from build123d import *

# Parameters (mm, degrees)
SKETCH1_R           = 14.9
BOSS_EXTRUDE1_DEPTH = 3
SKETCH2_R           = 7
CUT_EXTRUDE1_DEPTH  = 22.28426649
SKETCH3_R           = 14.9
SKETCH3_R_2         = 10.5
BOSS_EXTRUDE2_DEPTH = 3.5
CHAMFER1_SIZE       = 1
SKETCH4_R           = 1.75
CUT_EXTRUDE2_DEPTH  = 4
BOSS_EXTRUDE3_START = 2
SKETCH5_R           = 14.9
SKETCH5_R_2         = 10.5
SKETCH5_R_3         = 1.75
BOSS_EXTRUDE3_DEPTH = 2


with BuildPart() as part:
    # Sketch1 → Boss-Extrude1 (new body)
    with BuildSketch(Plane(origin=(0, 0, 0), x_dir=(-1, 0, 0), z_dir=(0, 1, 0))):
        with Locations(Location((0, 0, 0), (0, 0, 90))):
            Circle(SKETCH1_R)
    extrude(amount=BOSS_EXTRUDE1_DEPTH)

    # Sketch2 → Cut-Extrude1 (cut, through all)
    with BuildSketch(Plane(origin=(0, 3, 0), x_dir=(-1, 0, 0), z_dir=(0, 1, 0))):
        with Locations(Location((0, 0, 0), (0, 0, 90))):
            Circle(SKETCH2_R)
    extrude(amount=-CUT_EXTRUDE1_DEPTH, mode=Mode.SUBTRACT)

    # Sketch3 → Boss-Extrude2 (add)
    with BuildSketch(Plane(origin=(0, 3, 0), x_dir=(-1, 0, 0), z_dir=(0, 1, 0))):
        with Locations(Location((0, 0, 0), (0, 0, 90))):
            Circle(SKETCH3_R)
        with Locations(Location((0, 0, 0), (0, 0, 90))):
            Circle(SKETCH3_R_2, mode=Mode.SUBTRACT)
    extrude(amount=BOSS_EXTRUDE2_DEPTH)

    # Chamfer1
    chamfer1_edges = [part.edges().sort_by_distance(p)[0] for p in [
        (0, 0, -14.9),
        (0, 0, -7),
        (0, 3, -7),
    ]]
    chamfer(chamfer1_edges, length=CHAMFER1_SIZE)

    # Sketch4 → Cut-Extrude2 (cut)
    with BuildSketch(Plane(origin=(0, 6.5, 0), x_dir=(-1, 0, 0), z_dir=(0, 1, 0))):
        with Locations(Location((-12.7, 0, 0), (0, 0, 90))):
            Circle(SKETCH4_R)
        with Locations(Location((-0.075, 12.7, 0), (0, 0, 90))):
            Circle(SKETCH4_R)
        with Locations(Location((12.625, 0.075, 0), (0, 0, 90))):
            Circle(SKETCH4_R)
        with Locations(Location((0, -12.625, 0), (0, 0, 90))):
            Circle(SKETCH4_R)
    extrude(amount=-CUT_EXTRUDE2_DEPTH, mode=Mode.SUBTRACT)

    # Sketch5 → Boss-Extrude3 (add)
    with BuildSketch(Plane(origin=(0, 6.5, 0), x_dir=(-1, 0, 0), z_dir=(0, 1, 0)).offset(BOSS_EXTRUDE3_START)):
        with Locations(Location((0, 0, 0), (0, 0, 90))):
            Circle(SKETCH5_R)
        with Locations(Location((0, 0, 0), (0, 0, 90))):
            Circle(SKETCH5_R_2, mode=Mode.SUBTRACT)
        with Locations(Location((0, -12.625, 0), (0, 0, 90))):
            Circle(SKETCH5_R_3, mode=Mode.SUBTRACT)
        with Locations(Location((12.625, 0.075, 0), (0, 0, 90))):
            Circle(SKETCH5_R_3, mode=Mode.SUBTRACT)
        with Locations(Location((-0.075, 12.7, 0), (0, 0, 90))):
            Circle(SKETCH5_R_3, mode=Mode.SUBTRACT)
        with Locations(Location((-12.7, 0, 0), (0, 0, 90))):
            Circle(SKETCH5_R_3, mode=Mode.SUBTRACT)
    extrude(amount=-BOSS_EXTRUDE3_DEPTH)


solid = part.part
Geometry: final body of the model. Coordinates: model frame, mm. A direction names the side the tool comes from. Round coordinates to 2 decimals unless told otherwise and drop trailing zeros. Order: outer loops, then holes, each group sorted by start corner. A loop starts at its lowest first (then second) coordinate and runs counter-clockwise, first axis right, second up. Notation, with made-up numbers: (40.25, 19) -> (67.25, 19) arc R17 cw to (67.25, 27) -> close; hole circle Ø11 at (72, 73.5). An arc over 180 degrees is marked (long way). Put each result on its own line as item: value. Start each with the question number.
Q1. First-contact query: pin 1 (11 mm diameter, centred on x = 0, z = 0, fed in from +Y); pin 2 (5.5 mm diameter, centred on x = 0.075, z = 12.7, fed in from +Y); pin 3 (3 mm diameter, centred on y = 3.5, z = -4.5, fed in from +X); pin 4 (3 mm diameter, centred on x = 0, z = -12.625, fed in from +Y). Flat tips, straight axial feed; report the tip coordinate or a pass-through.
Q2. Pull-direction query (X, two-part tool) for faces 3 (the cylindrical face through (-10.89, 5.54, -0.15)), 4 (the flat face through (6, 8.5, -9)), 5 (the cylindrical face through (-13.219, 4.802, 6.875)); classes: +X half, -X half, draft (parallel to the pull), parting line (faces both ways), or undercut.
Q3. Section A-A on z = 0. Return the cut outline in (x, y), and give its area (3 significant figures).
Q4. Line query: probe 1 along X at (y, z) = (5.25, 0); probe 2 along Y at (x, z) = (6, 7); probe 3 along Z at (x, y) = (4.25, 2.5). Output: solid intervals per line, ascending.
Q5. Section B-B on y = 8. Return the cut outline in (x, z) (3 decimals), and give its area (3 significant figures).
Q6. Reachability of faces 1 (the cylindrical face through (3.2, 5.8, 10)), 2 (the cylindrical face through (-6.834, 1.507, -1.517)) from +Z, -Z, +X, -X, +Y, -Y: full face, straight path, thin tool, end or side. Return the list, or none.
Ans:
1. pin 1: passes through
1. pin 2: stops at y = 8.5
1. pin 3: stops at x = 14.59
1. pin 4: stops at y = 2.5
2. face 3: undercut
2. face 4: draft
2. face 5: parting line
3. outline: (-14.9, 1) -> (-13.9, 0) -> (-8, 0) -> (-7, 1) -> (-7, 2) -> (-8, 3) -> (-10.5, 3) -> (-10.5, 8.5) -> (-10.88, 8.5) -> (-10.88, 2.5) -> (-14.37, 2.5) -> (-14.37, 8.5) -> (-14.9, 8.5) -> close; (7, 1) -> (8, 0) -> (13.9, 0) -> (14.9, 1) -> (14.9, 8.5) -> (14.45, 8.5) -> (14.45, 2.5) -> (10.95, 2.5) -> (10.95, 8.5) -> (10.5, 8.5) -> (10.5, 3) -> (8, 3) -> (7, 2) -> close
3. area: 50.8 mm2
4. probe 1: x = -14.9 to -14.37, -10.88 to -10.5, 10.5 to 10.95, 14.45 to 14.9
4. probe 2: y = 0 to 3
4. probe 3: z = -14.28 to -6.18, 6.18 to 14.28
5. outline: circle Ø29.8 at (0, 0); hole circle Ø3.5 at (-12.625, 0.075); hole circle Ø21 at (0, 0); hole circle Ø3.5 at (0, -12.625); hole circle Ø3.5 at (0.075, 12.7); hole circle Ø3.5 at (12.7, 0)
5. area: 313 mm2
6. face 1: +Y
6. face 2: +Y, -Y
